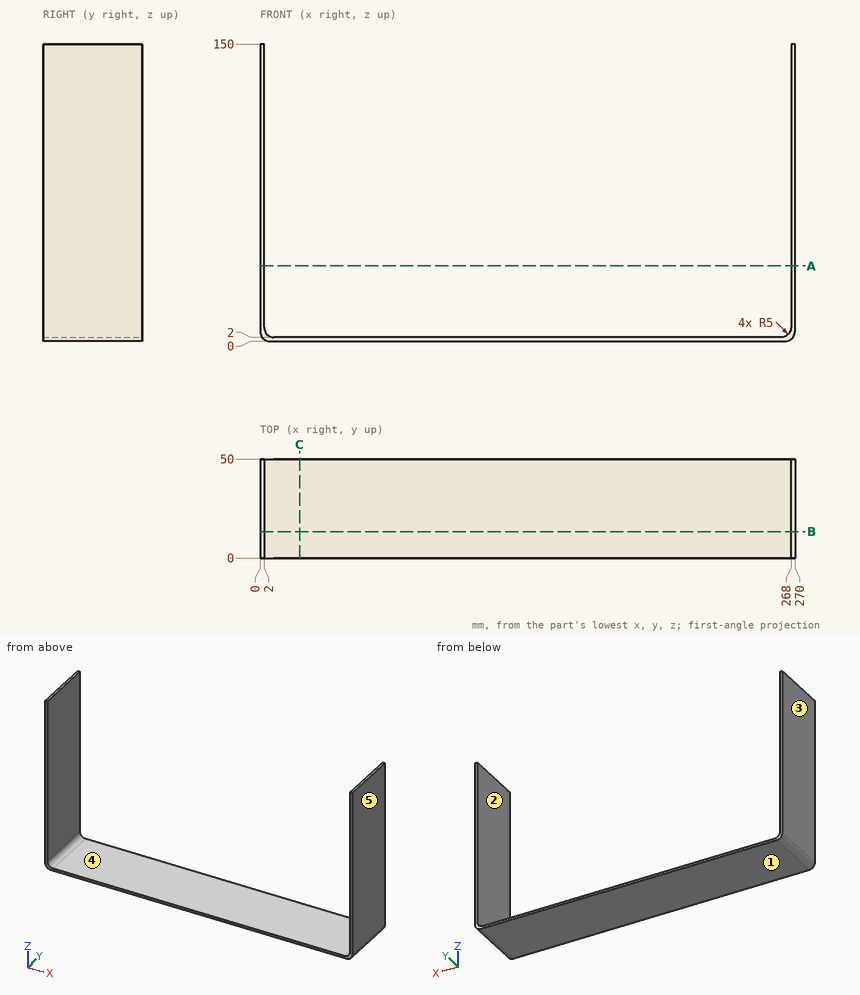
Geometry: see drawing. Coordinates: mm, zero at the bounding-box minimum. A direction names the side the tool comes from. Coordinates: 2 decimals unless noted, no trailing zeros. Loops run counter-clockwise (first coordinate to the right, second up) from the corner with the lowest first, then second, coordinate; pieces in that order, holes last. Notation, with made-up numbers: (80, 62.5) - (113, 62.5) arc R30 ccw to (113, 94.5) - close; hole circle Ø1 at (38.25, 76.25). An arc over 180 degrees is marked (long way). Answer in a Markdown table with one row per item.
(1) Cut plane B-B on y = 13.5. Output: boundary loops of the cut face in (x, z), plus the area to 3 significant figures.
Model answer:
| item | result |
|---|---|
| outline | (0, 5) arc R5 ccw to (5, 0) - (265, 0) arc R5 ccw to (270, 5) - (270, 150) - (268, 150) - (268, 7) arc R5 cw to (263, 2) - (7, 2) arc R5 cw to (2, 7) - (2, 150) - (0, 150) - close |
| area | 1,130 mm² |
(2) Cut plane A-A on z = 38. Output: boundary loops of the cut face in (x, y), plus the area to 3 significant figures.
Model answer:
| item | result |
|---|---|
| outline | (0, 0) - (2, 0) - (2, 50) - (0, 50) - close; (268, 0) - (270, 0) - (270, 50) - (268, 50) - close |
| area | 200 mm² |
(3) Pin query (flat end, axial travel): P1, Ø12, axis at x = 203.5, y = 6.5, coming from the +Z side. Return the tip coordinate at first contact, or that it passes through.
Model answer:
| item | result |
|---|---|
| P1 | stops at z = 2 |
(4) Material intervals for L1, parallel to X at y = 41, z = 10.5; L2, parallel to Z at x = 141, y = 42.5, sorted ascending. Write a range as from..to.
Model answer:
| item | result |
|---|---|
| L1 | x = 0..2, 268..270 |
| L2 | z = 0..2 |
(5) Mould query, pull axis X, two halves, no side actions, for the marked faces 1, 2 and 3. Classes: pulls with the +X half, pulls with the -X half, needs draft (parallel to the pull), parting line crosses it, or undercut.
Model answer:
| item | result |
|---|---|
| face 1 | needs draft |
| face 2 | undercut |
| face 3 | pulls with the -X half |
(6) Cut plane C-C on x = 20. Output: boundary loops of the cut face in (y, z).
Model answer:
| item | result |
|---|---|
| outline | (0, 0) - (50, 0) - (50, 2) - (0, 2) - close |
(7) Set-up query: the marked faces 4 and 5. Return all of +Z, -Z, +X, -X, +Y, -Y with unobstructed straight access to the full face (end or side cutting, diameter ignored); none if empty.
Model answer:
| item | result |
|---|---|
| face 4 | +Z, +Y, -Y |
| face 5 | +Z, -Z, +X, +Y, -Y |
